Source: CAD feature listing. Evaluate the final solid. Frame: model axes, mm. Give positions to 0.01 mm unless a question says otherwise; leave off trailing zeros. Order: outer loops, then holes, each group sorted by start corner. A loop starts at its lowest first (then second) coordinate and runs counter-clockwise, first axis right, second up. Notation, with made-up numbers: M -6,-6.75 L 22,-6.75 A28 cw 22,22.25 Z; hole C 47,-5 d9. An arc over 180 degrees is marked long. One line per question, with ' | ' between items. Start each with the question number.
from build123d import *

# Parameters (mm, degrees)
SKETCH1_R           = 17.4625
SKETCH1_R_2         = 3.175
SKETCH1_R_3         = 2.0193
SKETCH1_R_4         = 11.1125
SKETCH1_R_5         = 9.5885
SKETCH1_R_6         = 2.4892
BOSS_EXTRUDE1_DEPTH = 3.175


with BuildPart() as part:
    # Sketch1 → Boss-Extrude1 (new, symmetric)
    with BuildSketch(Plane.XY):
        with BuildLine():
            Line((-63.4492, 47.0662), (-63.4492, 6.387701907))
            ThreePointArc((-63.4492, 6.387701907), (-61.443306044, -0.347944705), (-56.079239896, -4.888797072))
            Line((-56.079239896, -4.888797072), (-10.832597323, -24.718009456))
            ThreePointArc((-10.832597323, -24.718009456), (-5.8974e-05, -26.9875), (10.832489293, -24.7180568))
            Line((10.832489293, -24.7180568), (56.079190612, -4.8890544))
            ThreePointArc((56.079190612, -4.8890544), (61.443291325, -0.348202956), (63.4492, 6.387466177))
            Line((63.4492, 6.387466177), (63.4492, 47.0662))
            ThreePointArc((63.4492, 47.0662), (54.559012129, 68.529012129), (33.0962, 77.4192))
            Line((33.0962, 77.4192), (-33.0962, 77.4192))
            ThreePointArc((-33.0962, 77.4192), (-54.559012129, 68.529012129), (-63.4492, 47.0662))
        make_face()
        Circle(SKETCH1_R, mode=Mode.SUBTRACT)
        with Locations((47.625, 0)):
            Circle(SKETCH1_R_2, mode=Mode.SUBTRACT)
        with Locations((-23.8125, 0)):
            Circle(SKETCH1_R_3, mode=Mode.SUBTRACT)
        with Locations((-47.625, 0)):
            Circle(SKETCH1_R_2, mode=Mode.SUBTRACT)
        with Locations((23.8125, 0)):
            Circle(SKETCH1_R_3, mode=Mode.SUBTRACT)
        with Locations((0, 47.0662)):
            Circle(SKETCH1_R_4, mode=Mode.SUBTRACT)
        with Locations((33.0962, 47.0662)):
            Circle(SKETCH1_R_5, mode=Mode.SUBTRACT)
        with Locations((-33.0962, 47.0662)):
            Circle(SKETCH1_R_5, mode=Mode.SUBTRACT)
        with Locations((-25.940193056, 71.43732153)):
            Circle(SKETCH1_R_6, mode=Mode.SUBTRACT)
        with Locations((-40.252206944, 22.69507847)):
            Circle(SKETCH1_R_6, mode=Mode.SUBTRACT)
        with Locations((40.945231657, 22.909364486)):
            Circle(SKETCH1_R_6, mode=Mode.SUBTRACT)
        with Locations((25.247168343, 71.223035514)):
            Circle(SKETCH1_R_6, mode=Mode.SUBTRACT)
    extrude(amount=BOSS_EXTRUDE1_DEPTH, both=True)


solid = part.part
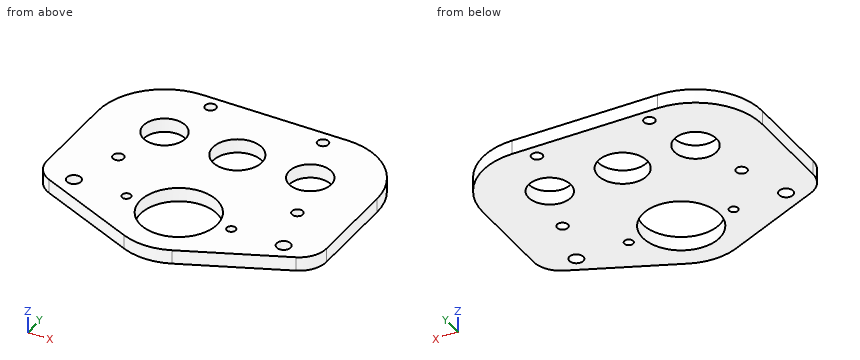
Item 1: Line query: line 1 (X direction, y = 72, z = -2.25); line 2 (X direction, y = 53, z = 1.5); line 3 (Y direction, x = -8, z = -0.5). Output: solid intervals per line, ascending.
Item 2: Cut plane A-A on x = 0. Return the cut outline in (y, z) (1 decimal), and give its area (3 significant figures).
Item 3: Cut plane D-D on x = 34.5. Return the cut outline in (y, z) (3 decimals), and give its area (3 significant figures).
Item 4: Pin query (flat end, axial travel): pin 1 Ø11.5 at (x, y) = (33.1, 47.07) entering from +Z; pin 2 Ø1 at (x, z) = (-24, -1.5) entering from -Y. Return the tip coordinate at first contact, or that it passes through.
Item 5: Cut plane B-B on y = -16. Return the cut outline in (x, z) (1 decimal).
Item 6: Cut plane C-C on y = 0. Count the separate pieces of the cut face and the enclosed holes in it, and give its area (3 significant figures).
Results are:
1) line 1: x = -50.41 to -28.36, -23.52 to 22.88, 27.61 to 50.41 | line 2: x = -62.86 to -40.63, -25.56 to -9.4, 9.4 to 25.56, 40.63 to 62.86 | line 3: y = -25.77 to -15.52, 15.52 to 39.35, 54.78 to 77.42
2) outline: M -27,-3.2 L -17.5,-3.2 L -17.5,3.2 L -27,3.2 Z; M 17.5,-3.2 L 36,-3.2 L 36,3.2 L 17.5,3.2 Z; M 58.2,-3.2 L 77.4,-3.2 L 77.4,3.2 L 58.2,3.2 Z | area: 300 mm2
3) outline: M -14.346,-3.175 L 37.581,-3.175 L 37.581,3.175 L -14.346,3.175 Z; M 56.551,-3.175 L 77.387,-3.175 L 77.387,3.175 L 56.551,3.175 Z | area: 462 mm2
4) pin 1: passes through | pin 2: stops at y = -19.17
5) outline: M -30.7,-3.2 L -7,-3.2 L -7,3.2 L -30.7,3.2 Z; M 7,-3.2 L 30.7,-3.2 L 30.7,3.2 L 7,3.2 Z
6) separate pieces: 6 | enclosed holes: 0 | area: 429 mm2
